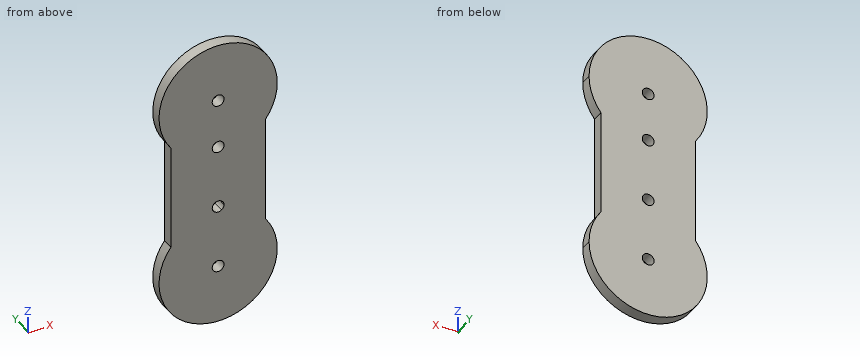
```python
from build123d import *

# Parameters (mm, degrees)
F0_R     = 2.5
F1_DEPTH = 5


with BuildPart() as f1:
    # F0 (on Front) → F1 (new body)
    with BuildSketch(Plane.XZ):
        with BuildLine():
            ThreePointArc((20, 32.8825393335), (23.7170824513, 39.9768451831), (25, 47.8825393335))
            ThreePointArc((25, 47.8825393335), (-7.9056941504, 71.5996217848), (-20, 32.8825393335))
            Line((-20, 32.8825393335), (20, 32.8825393335))
        make_face()
        with Locations((0, 47.8825393335)):
            Circle(F0_R, mode=Mode.SUBTRACT)
        with BuildLine():
            Line((20, 32.8825393335), (-20, 32.8825393335))
            ThreePointArc((-20, 32.8825393335), (0, 22.8825393335), (20, 32.8825393335))
        make_face()
        with Locations((0, 26.8825393335)):
            Circle(F0_R, mode=Mode.SUBTRACT)
        with BuildLine():
            ThreePointArc((20, 32.8825393335), (0, 22.8825393335), (-20, 32.8825393335))
            Line((-20, 32.8825393335), (-20, -12.1174606665))
            ThreePointArc((-20, -12.1174606665), (-11.821177666, -5.0888483954), (-1.4427741411, -2.1591273332))
            ThreePointArc((-1.4427741411, -2.1591273332), (-1.1495791942, 2.1025545759), (2.5, -0.1174606665))
            ThreePointArc((2.5, -0.1174606665), (2.2200152424, -1.2670398606), (1.4427741411, -2.1591273332))
            ThreePointArc((1.4427741411, -2.1591273332), (11.821177666, -5.0888483954), (20, -12.1174606665))
            Line((20, -12.1174606665), (20, 32.8825393335))
        make_face()
        with BuildLine():
            Line((20, -12.1174606665), (-20, -12.1174606665))
            ThreePointArc((-20, -12.1174606665), (-7.9056941504, -50.8345431177), (25, -27.1174606665))
            ThreePointArc((25, -27.1174606665), (23.7170824513, -19.2117665161), (20, -12.1174606665))
        make_face()
        with Locations((0, -27.1174606665)):
            Circle(F0_R, mode=Mode.SUBTRACT)
        with BuildLine():
            ThreePointArc((-1.4427741411, -2.1591273332), (-11.821177666, -5.0888483954), (-20, -12.1174606665))
            Line((-20, -12.1174606665), (20, -12.1174606665))
            ThreePointArc((20, -12.1174606665), (11.821177666, -5.0888483954), (1.4427741411, -2.1591273332))
            ThreePointArc((1.4427741411, -2.1591273332), (0, -2.6174606665), (-1.4427741411, -2.1591273332))
        make_face()
    extrude(amount=F1_DEPTH)


solid = f1.part
```
Read the model definition and answer for the solid it produces. Units are mm, in the model's axes. Round coordinates to 2 decimals unless told otherwise and drop trailing zeros. Write each loop counter-clockwise with the first axis right and the second up, starting at its lowest first coordinate (ties: lowest second). Pieces come first, ordered by that corner, then holes. Notation, with made-up numbers: (34.5, -25.75) - (61.5, -25.75) arc R26 cw to (61.5, -5.75) - close; hole circle Ø8 at (-18.75, -23.75). An arc over 180 degrees is marked (long way). One line per item, written item: value.
Q1. Find section D-D (x = -14). Determine the outline of the cut face in (y, z).
The answers:
outline: (-5, -47.83) - (0, -47.83) - (0, 68.59) - (-5, 68.59) - close
Q2. Find section A-A (x = 0). Determine the outline of the cut face in (y, z), and give its area (3 significant figures).
The answers:
outline: (-5, -52.12) - (0, -52.12) - (0, -29.62) - (-5, -29.62) - close; (-5, -24.62) - (0, -24.62) - (0, -2.62) - (-5, -2.62) - close; (-5, 2.38) - (0, 2.38) - (0, 24.38) - (-5, 24.38) - close; (-5, 29.38) - (0, 29.38) - (0, 45.38) - (-5, 45.38) - close; (-5, 50.38) - (0, 50.38) - (0, 72.88) - (-5, 72.88) - close
area: 525 mm2
Q3. Find section C-C (z = 3.5). Determine the outline of the cut face in (x, y).
The answers:
outline: (-20, -5) - (20, -5) - (20, 0) - (-20, 0) - close
Q4. Find section B-B (y = -2.3). Determine the outline of the cut face in (x, z).
The answers:
outline: (-20, -12.12) arc R25 ccw (long way) to (20, -12.12) - (20, 32.88) arc R25 ccw (long way) to (-20, 32.88) - close; hole circle Ø5 at (0, -27.12); hole circle Ø5 at (0, -0.12); hole circle Ø5 at (0, 26.88); hole circle Ø5 at (0, 47.88)
Q5. Straight lines are drawn through the part: line 1 (X direction, y = -2.85, z = 3); line 2 (Z direction, x = -1, y = -1.75); line 3 (X direction, y = -0.85, z = 47.5). For each, find the intervals that lie inside material, in ascending order. Write a range as from..to.
The answers:
line 1: x = -20..20
line 2: z = -52.1..-29.41, -24.83..-2.41, 2.17..24.59, 29.17..45.59, 50.17..72.86
line 3: x = -25..-2.47, 2.47..25
Q6. Each of these flat-tipped pins is pushed along its axis until it touches: P1, Ø2.5, axis at y = -3.5, z = 6, coming from the +X side; P2, Ø4, axis at x = 0, z = -27.12, coming from the -Y side; P3, Ø3, axis at x = 1.5, y = -3, coming from the -Z side. Where does it stop, or does it pass through?
The answers:
P1: stops at x = 20
P2: passes through
P3: stops at z = -52.12
